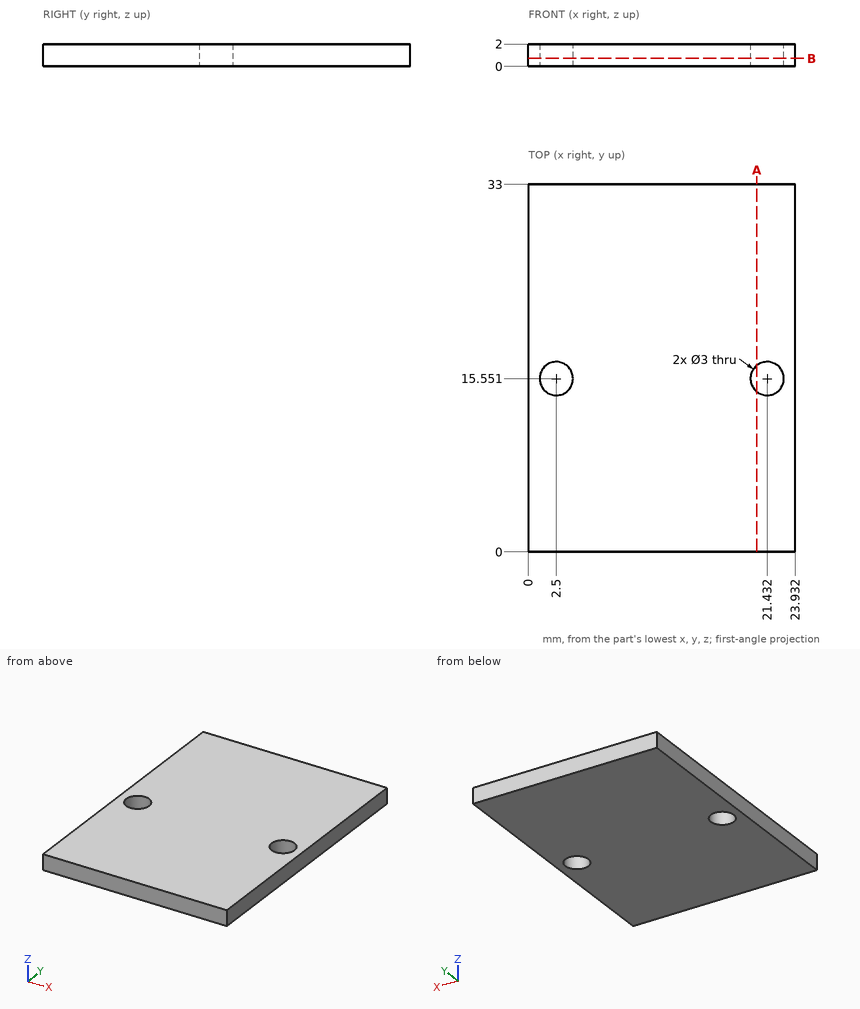
Source: three-view drawing plus pictorial views. Frame: mm from the lowest corner of the part. Round coordinates to 2 decimals unless told otherwise and drop trailing zeros. Loops run counter-clockwise (first coordinate to the right, second up) from the corner with the lowest first, then second, coordinate; pieces in that order, holes last.
Q1. Pin query (flat end, axial travel): P1, Ø5, axis at x = 21.432, y = 15.551, coming from the -Z side. Return the tip coordinate at first contact, or that it passes through.
Q2. Section A-A on x = 20.5. Return loops of the section in (y, z), plus the area to 3 significant figures.
Q3. Section B-B on z = 0.7. Return loops of the section in (x, y), plus the area to 3 significant figures.
Q4. Material intervals for L1, parallel to Y at x = 2.5, z = 1.4, sorted ascending.
Evaluation:
1. P1: stops at z = 0
2. outline: (0, 0) - (14.38, 0) - (14.38, 2) - (0, 2) - close; (16.73, 0) - (33, 0) - (33, 2) - (16.73, 2) - close
2. area: 61.3 mm2
3. outline: (0, 0) - (23.93, 0) - (23.93, 33) - (0, 33) - close; hole circle Ø3 at (2.5, 15.55); hole circle Ø3 at (21.43, 15.55)
3. area: 776 mm2
4. L1: y = 0 to 14.05, 17.05 to 33
